Input: part model. Units: mm. Frame: model coordinates. Coordinates: 2 decimals unless noted, no trailing zeros. Order: outer loops, then holes, each group sorted by start corner. A loop starts at its lowest first (then second) coordinate and runs counter-clockwise, first axis right, second up. Notation, with made-up numbers: M -23.75,71 L 8.25,71 A24 ccw 8.25,98 Z; hole C 87,65 d1. An arc over 180 degrees is marked long. Answer in a Markdown table with one row per item.
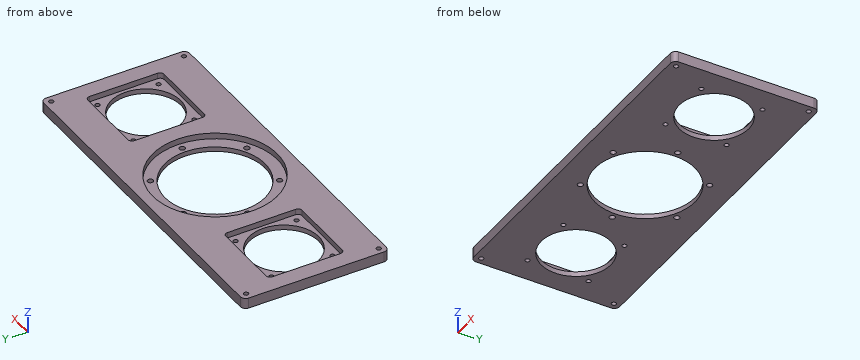
from build123d import *

# Parameters (mm, degrees)
SKETCH_W           = 260
SKETCH_H           = 110
SKETCH_R           = 37.75
SKETCH_R_2         = 26.25
SKETCH_R_3         = 1.75
PAD_DEPTH          = 8
SKETCH001_R        = 2.1
POCKET_DEPTH       = 8
POLARPATTERN_COUNT = 6
SKETCH002_R        = 47
SKETCH002_R_2      = 1.75
POCKET001_DEPTH    = 4.5
SKETCH003_R        = 26.25
POCKET002_DEPTH    = 4.3
SKETCH004_R        = 1.75
POCKET003_DEPTH    = 8
FILLET002_R        = 4


with BuildPart() as part:
    # Sketch → Pad (new body)
    with BuildSketch(Plane.XY):
        Rectangle(SKETCH_W, SKETCH_H)
        Circle(SKETCH_R, mode=Mode.SUBTRACT)
        with Locations((88.5, 0)):
            Circle(SKETCH_R_2, mode=Mode.SUBTRACT)
        with Locations((-88.5, 0)):
            Circle(SKETCH_R_2, mode=Mode.SUBTRACT)
        with Locations((111.516326, -23.016326)):
            Circle(SKETCH_R_3, mode=Mode.SUBTRACT)
        with Locations((111.516326, 23.016326)):
            Circle(SKETCH_R_3, mode=Mode.SUBTRACT)
        with Locations((65.483674, 23.016326)):
            Circle(SKETCH_R_3, mode=Mode.SUBTRACT)
        with Locations((65.483674, -23.016326)):
            Circle(SKETCH_R_3, mode=Mode.SUBTRACT)
        with Locations((-111.516326, 23.016326)):
            Circle(SKETCH_R_3, mode=Mode.SUBTRACT)
        with Locations((-65.483674, 23.016326)):
            Circle(SKETCH_R_3, mode=Mode.SUBTRACT)
        with Locations((-65.483674, -23.016326)):
            Circle(SKETCH_R_3, mode=Mode.SUBTRACT)
        with Locations((-111.516326, -23.016326)):
            Circle(SKETCH_R_3, mode=Mode.SUBTRACT)
    extrude(amount=PAD_DEPTH)

    # Sketch001 (on Face17 of Pad) → Pocket (cut)
    with BuildSketch(Plane.XY.offset(8)):
        with Locations((42, 0)):
            Circle(SKETCH001_R)
    pocket = extrude(amount=-POCKET_DEPTH, mode=Mode.SUBTRACT)

    # PolarPattern: Pocket ×6 about axis
    polarpattern_axis = Axis((0, 0, 8), (0, 0, 1))
    for i in range(1, POLARPATTERN_COUNT):
        add(pocket.rotate(polarpattern_axis, i * 360 / POLARPATTERN_COUNT), mode=Mode.SUBTRACT)

    # Sketch002 (on Face5 of PolarPattern) → Pocket001 (cut)
    with BuildSketch(Plane.XY.offset(8)):
        Circle(SKETCH002_R)
        Circle(SKETCH002_R_2, mode=Mode.SUBTRACT)
    extrude(amount=-POCKET001_DEPTH, mode=Mode.SUBTRACT)

    # Sketch003 (on Face5 of Pocket001) → Pocket002 (cut)
    with BuildSketch(Plane.XY.offset(8)):
        with BuildLine():
            Line((-114.25, 28.75), (-62.75, 28.75))
            ThreePointArc((-59.75, 25.75), (-60.62868, 27.87132), (-62.75, 28.75))
            Line((-59.75, 25.75), (-59.75, -25.75))
            ThreePointArc((-62.75, -28.75), (-60.62868, -27.87132), (-59.75, -25.75))
            Line((-62.75, -28.75), (-114.25, -28.75))
            ThreePointArc((-117.25, -25.75), (-116.37132, -27.87132), (-114.25, -28.75))
            Line((-117.25, -25.75), (-117.25, 25.75))
            ThreePointArc((-114.25, 28.75), (-116.37132, 27.87132), (-117.25, 25.75))
        make_face()
        with Locations((-88.5, 0)):
            Circle(SKETCH003_R, mode=Mode.SUBTRACT)
        with BuildLine():
            Line((62.75, 28.75), (114.25, 28.75))
            ThreePointArc((117.25, 25.75), (116.37132, 27.87132), (114.25, 28.75))
            Line((117.25, 25.75), (117.25, -25.75))
            ThreePointArc((114.25, -28.75), (116.37132, -27.87132), (117.25, -25.75))
            Line((114.25, -28.75), (62.75, -28.75))
            ThreePointArc((59.75, -25.75), (60.62868, -27.87132), (62.75, -28.75))
            Line((59.75, -25.75), (59.75, 25.75))
            ThreePointArc((62.75, 28.75), (60.62868, 27.87132), (59.75, 25.75))
        make_face()
        with Locations((88.5, 0)):
            Circle(SKETCH003_R, mode=Mode.SUBTRACT)
    extrude(amount=-POCKET002_DEPTH, mode=Mode.SUBTRACT)

    # Sketch004 (on Face5 of Pocket002) → Pocket003 (cut)
    with BuildSketch(Plane.XY.offset(8)):
        with Locations((-125, 50)):
            Circle(SKETCH004_R)
        with Locations((-125, -50)):
            Circle(SKETCH004_R)
        with Locations((125, -50)):
            Circle(SKETCH004_R)
        with Locations((125, 50)):
            Circle(SKETCH004_R)
    extrude(amount=-POCKET003_DEPTH, mode=Mode.SUBTRACT)

    # Fillet002
    fillet002_edges = [part.edges().sort_by_distance(p)[0] for p in [
        (130, -55, 4),
        (-130, -55, 4),
        (-130, 55, 4),
        (130, 55, 4),
    ]]
    fillet(fillet002_edges, radius=FILLET002_R)


solid = part.part
1) Cut plane A-A, the plane z = 5.25. State how many separate pieces and enclosed holes the cut face has, and give its area (3 significant figures).
Resolved:
| item | result |
|---|---|
| separate pieces | 1 |
| enclosed holes | 7 |
| area | 15,000 mm2 |
2) Contact query for flat-ended pins moving along their axis: pin 1 (3.5 mm diameter, centred on x = -21, y = 36.37, fed in from -Z); pin 2 (5 mm diameter, centred on x = -21, y = -36.37, fed in from +Z); pin 3 (4.5 mm diameter, centred on x = -65.48, y = -23.02, fed in from +Z). Output: stop coordinate, or through.
Resolved:
| item | result |
|---|---|
| pin 1 | passes through |
| pin 2 | stops at z = 3.5 |
| pin 3 | stops at z = 3.7 |
3) Cut plane C-C, the plane y = -17. Output: boundary loops of the cut face in (x, z), and give its area (3 significant figures).
Resolved:
| item | result |
|---|---|
| outline | M -130,0 L -108.5,0 L -108.5,3.7 L -117.25,3.7 L -117.25,8 L -130,8 Z; M -68.5,0 L -33.71,0 L -33.71,3.5 L -43.82,3.5 L -43.82,8 L -59.75,8 L -59.75,3.7 L -68.5,3.7 Z; M 33.71,0 L 68.5,0 L 68.5,3.7 L 59.75,3.7 L 59.75,8 L 43.82,8 L 43.82,3.5 L 33.71,3.5 Z; M 108.5,0 L 130,0 L 130,8 L 117.25,8 L 117.25,3.7 L 108.5,3.7 Z |
| area | 659 mm2 |
4) Cut plane D-D, the plane x = 12.5. Output: boundary loops of the cut face in (y, z).
Resolved:
| item | result |
|---|---|
| outline | M -55,0 L -35.62,0 L -35.62,3.5 L -45.31,3.5 L -45.31,8 L -55,8 Z; M 35.62,0 L 55,0 L 55,8 L 45.31,8 L 45.31,3.5 L 35.62,3.5 Z |
5) Cut plane B-B, the plane x = -87. Output: boundary loops of the cut face in (y, z), and give its area (3 significant figures).
Resolved:
| item | result |
|---|---|
| outline | M -55,0 L -26.21,0 L -26.21,3.7 L -28.75,3.7 L -28.75,8 L -55,8 Z; M 26.21,0 L 55,0 L 55,8 L 28.75,8 L 28.75,3.7 L 26.21,3.7 Z |
| area | 439 mm2 |
6) Material intervals for probe 1 along Y at (x, z) = (-88.5, 2.9); probe 2 along Y at (x, z) = (-125, 2.25); probe 3 along X at (y, z) = (-24, 5.75), sorted ascending.
Resolved:
| item | result |
|---|---|
| probe 1 | y = -55 to -26.25, 26.25 to 55 |
| probe 2 | y = -55 to -51.75, -48.25 to 48.25, 51.75 to 55 |
| probe 3 | x = -130 to -117.25, -59.75 to -40.41, 40.41 to 59.75, 117.25 to 130 |
